```python
from build123d import *

# Parameters (mm, degrees)
SKETCH1_R           = 4
BOSS_EXTRUDE1_DEPTH = 60.96
FILLET2_R           = 0.254
SKETCH2_W           = 8
SKETCH2_H           = 12.7
CUT_EXTRUDE1_DEPTH  = 2.38125


with BuildPart() as part:
    # Sketch1 → Boss-Extrude1 (new body)
    with BuildSketch(Plane.XY):
        Circle(SKETCH1_R)
    extrude(amount=BOSS_EXTRUDE1_DEPTH)

    # Fillet2
    fillet2_edges = [part.edges().sort_by_distance(p)[0] for p in [
        (-4, 0, 0),
        (-4, 0, 60.96),
    ]]
    fillet(fillet2_edges, radius=FILLET2_R)

    # Sketch2 → Cut-Extrude1 (cut)
    with BuildSketch(Plane(origin=(0, 4, 0), x_dir=(1, 0, 0), z_dir=(0, 1, 0))):
        with Locations((0, -6.35)):
            Rectangle(SKETCH2_W, SKETCH2_H)
    extrude(amount=-CUT_EXTRUDE1_DEPTH, mode=Mode.SUBTRACT)


solid = part.part
```
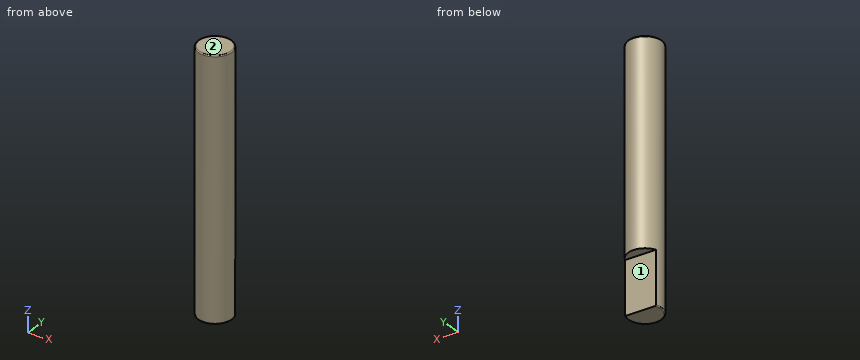
The model under review builds one solid part; all positions refer to its coordinate system, in mm. Face numbers are marked on the shaded views. A direction names the side the tool comes from. Give positions to 0.01 mm unless a question says otherwise; leave off trailing zeros. Loops run counter-clockwise (first coordinate to the right, second up) from the corner with the lowest first, then second, coordinate; pieces in that order, holes last. Notation, with made-up numbers: (-8.5, -14) - (11.5, -14) arc R13 cw to (11.5, -10) - close; hole circle Ø8 at (-1.5, 27.25). An arc over 180 degrees is marked (long way). Answer as a JSON object with one key per item and string values.
Q1. Add section B-B on z = 29. State the section outline as (x, y) points, plus the area to 3 significant figures.
Worked out:
{"outline": "circle Ø8 at (0, 0)", "area": "50.3 mm^2"}
Q2. To check wall thickness, follow line 1 along Z through (x, y) = (2, 3); line 2 along Y through (x, z) = (-0.25, 6.5); line 3 along Y through (x, z) = (0.25, 44.5). State the ranges of each line that lie inside material, in increasing order.
Worked out:
{"line 1": "z = 12.7 to 60.96", "line 2": "y = -3.99 to 1.62", "line 3": "y = -3.99 to 3.99"}
Q3. Add section A-A on x = 0. State the section outline as (y, z) points, plus the area to 3 significant figures.
Worked out:
{"outline": "(-4, 0.25) arc R0.25 ccw to (-3.75, 0) - (1.62, 0) - (1.62, 12.7) - (4, 12.7) - (4, 60.71) arc R0.25 ccw to (3.75, 60.96) - (-3.75, 60.96) arc R0.25 ccw to (-4, 60.71) - close", "area": "457 mm^2"}
Q4. For the marked faces 1 and 2, list the 3-axis set-ups (+Z, -Z, +X, -X, +Y, -Y) from which the entire face can be reached by the end or side of a thin tool; tool diameter is ignored.
Worked out:
{"face 1": "-Z, +X, -X, +Y", "face 2": "+Z, +X, -X, +Y, -Y"}
Q5. Insertion check: pin 1 (1.5 mm diameter, centred on y = -1, z = 15, fed in from -X); pin 2 (1.5 mm diameter, centred on x = 1.5, z = 10, fed in from -Y); pin 3 (1.2 mm diameter, centred on x = 0, y = 3, fed in from -Z). Each pin has a flat end and moves straight along its axis. Give the tip position at first contact, or say it passes through.
Worked out:
{"pin 1": "stops at x = -3.99", "pin 2": "stops at y = -3.93", "pin 3": "stops at z = 12.7"}
